```python
from build123d import *

# Parameters (mm, degrees)
ESQUISSE1_R             = 175
BOSS_EXTRU_1_DEPTH      = 5
ESQUISSE2_R             = 4.7
ENL_V_MAT_EXTRU_1_DEPTH = 5
LEDS_BOUT_TIRETTE_R     = 10.7
LEDS_BOUT_TIRETTE_R_2   = 6.25
LEDS_BOUT_TIRETTE_R_3   = 4
LEDS_BOUT_TIRETTE_R_4   = 5
LEDS_BOUT_TIRETTE_R_5   = 7.5
ENL_V_MAT_EXTRU_2_DEPTH = 10


with BuildPart() as part:
    # Esquisse1 → Boss.-Extru.1 (new body)
    with BuildSketch(Plane.XY):
        Circle(ESQUISSE1_R)
    extrude(amount=BOSS_EXTRU_1_DEPTH)

    # Esquisse2 → Enlèv. mat.-Extru.1 (cut)
    with BuildSketch(Plane(origin=(0, 0, 0), x_dir=(-1, 0, 0), z_dir=(0, 0, -1))):
        with Locations((-18.220426897, 85.887612711)):
            Circle(ESQUISSE2_R)
        with Locations((40.460378836, 115.887612711)):
            Circle(ESQUISSE2_R)
        with Locations((-65.270641029, -58.723158916)):
            Circle(ESQUISSE2_R)
        with Locations((-120.59180601, -22.904090436)):
            Circle(ESQUISSE2_R)
        Polygon((26.7795731, 95.88761271), (38.263317053, 161.015161015), (68.550112498, 161.015161015), (68.550112498, 190.246123658), (-94.990966298, 190.246123658), (-94.990966298, 161.015161015), (-64.704170853, 161.015161015), (-53.2204269, 95.88761271), align=None)
        Polygon((-96.430895065, -24.752015748), (-158.57487836, -47.370575906), (-173.718276082, -21.141441652), (-199.033032308, -35.756922974), (-117.262492911, -177.387651773), (-91.947736684, -162.772170451), (-107.091134406, -136.543036197), (-56.430895065, -94.034048051), align=None)
    extrude(amount=-ENL_V_MAT_EXTRU_1_DEPTH, mode=Mode.SUBTRACT)

    # Leds, bout., tirette → Enlèv. mat.-Extru.2 (cut)
    with BuildSketch(Plane.XY.offset(5)):
        with Locations((-90.932667397, -52.5)):
            Circle(LEDS_BOUT_TIRETTE_R)
        with Locations((-96.24355653, -113.301270189)):
            Circle(LEDS_BOUT_TIRETTE_R_2)
        with Locations((-136.24355653, -44.019237886)):
            Circle(LEDS_BOUT_TIRETTE_R_3)
        with Locations((-106.24355653, -95.980762114)):
            Circle(LEDS_BOUT_TIRETTE_R_3)
        with Locations((-146.064064606, -67.009618943)):
            Circle(LEDS_BOUT_TIRETTE_R_3)
        with Locations((-131.064064606, -92.990381057)):
            Circle(LEDS_BOUT_TIRETTE_R_4)
        with Locations((-146.24355653, -26.698729811)):
            Circle(LEDS_BOUT_TIRETTE_R_5)
        with BuildLine():
            Line((-118.94355653, -73.983716857), (-125.222240707, -77.608716857))
            Line((-125.222240707, -77.608716857), (-129.822240707, -69.641283143))
            Line((-129.822240707, -69.641283143), (-123.54355653, -66.016283143))
            ThreePointArc((-123.54355653, -66.016283143), (-117.259839672, -67.7), (-118.94355653, -73.983716857))
        make_face()
        Polygon((-126.003175473, -31.756098166), (-100.02241336, -16.756098166), (-94.52241336, -26.282377607), (-120.503175473, -41.282377607), align=None)
        Polygon((-96.003175473, -83.717622393), (-70.02241336, -68.717622393), (-64.52241336, -78.243901834), (-90.503175473, -93.243901834), align=None)
    extrude(amount=-ENL_V_MAT_EXTRU_2_DEPTH, mode=Mode.SUBTRACT)


solid = part.part
```
Input: part model. Units: mm. Frame: model coordinates. A direction names the side the tool comes from. Round coordinates to 2 decimals unless told otherwise and drop trailing zeros. Loops run counter-clockwise (first coordinate to the right, second up) from the corner with the lowest first, then second, coordinate; pieces in that order, holes last. Notation, with made-up numbers: (75.25, -16.75) -> (91.25, -16.75) arc R24 ccw to (91.25, -0.75) -> close; hole circle Ø3 at (-12, 38). An arc over 180 degrees is marked (long way). Write each question's results on one line, items separated by ' | '.
1. Section C-C (z = 4.15). State how many separate pieces and enclosed holes the cut face has, and give its area (3 significant figures).
Geometry results:
separate pieces: 1 | enclosed holes: 14 | area: 79,800 mm2
2. Mould query, pull axis X, two halves, no side actions, for faces 4 (the face through (-77.33, -85.64, 2.54)), 5 (the face through (-2, -5, 0)), 6 (the face through (166.04, -34.44, 2.46)), 7 (the face through (-136.06, -92.77, 2.54)). Classes: +X half, -X half, draft (parallel to the pull), parting line (faces both ways), or undercut.
Geometry results:
face 4: undercut | face 5: draft | face 6: +X half | face 7: undercut
3. Section A-A (x = 75.5). Return loops of the section in (y, z).
Geometry results:
outline: (-157.88, 0) -> (-110.03, 0) -> (-110.03, 5) -> (-157.88, 5) -> close; (-61.01, 0) -> (157.88, 0) -> (157.88, 5) -> (-61.01, 5) -> close
4. Section D-D (x = -56.5). Return loops of the section in (y, z).
Geometry results:
outline: (-165.63, 0) -> (161.02, 0) -> (161.02, 5) -> (-165.63, 5) -> close
5. First-contact query: P1, Ø1.5, axis at x = 37, z = 3, coming from the -Y side; P2, Ø10, axis at x = -96.24, y = -113.3, coming from the +Z side; P3, Ø1.5, axis at x = 0.5, z = 2.5, coming from the +Y side; P4, Ø3, axis at x = 131, z = 4.5, coming from the +Y side. Flat tips, straight axial feed; report the tip coordinate or a pass-through.
Geometry results:
P1: y = -171.2 | P2: through | P3: y = 95.89 | P4: y = 117.71
6. Section B-B (x = 0). Return loops of the section in (y, z), and give its area (3 significant figures).
Geometry results:
outline: (-175, 0) -> (95.89, 0) -> (95.89, 5) -> (-175, 5) -> close | area: 1,350 mm2
7. Ray query, line 1 (X direction, y = -72.5, z = 2.95); line 2 (Y direction, x = 65, z = 3.4); line 3 (Y direction, x = -68.5, z = 1.8). Return the intervals inside material, ascending. Write a range as from..to.
Geometry results:
line 1: -159.28..-128.17, -117.38..-76.57, -67.84..68.86 | line 2: -162.48..-101.22, -79.19..-63.42, -54.03..161.02 | line 3: -161.04..-80.54, -71.35..161.02
8. Set-up query: faces 1 (the face through (-2, -5, 5)), 2 (the face through (-107.331, -33.677, 2.535)), 3 (the face through (59.043, 128.907, 2.465)). Return all of +Z, -Z, +X, -X, +Y, -Y with unobstructed straight access to the full face (end or side cutting, diameter ignored); none if empty.
Geometry results:
face 1: +Z, +X, -X, +Y, -Y | face 2: +Z, -Z | face 3: +Z, -Z, +Y
